Input: part model. Units: mm. Frame: model coordinates. A direction names the side the tool comes from. Round coordinates to 2 decimals unless told otherwise and drop trailing zeros. Order: outer loops, then holes, each group sorted by start corner. A loop starts at its lowest first (then second) coordinate and runs counter-clockwise, first axis right, second up.
Item 1: Mould query, pull axis Z, two halves, no side actions, for faces 1 (the cylindrical face through (-1.984, 5.423, -1.521)), 2 (the flat face through (2, 0, -2)), 3 (the cylindrical face through (2.99, 18.45, -1.43)), 4 (the cylindrical face through (-0.867, 11.832, 3.905)). Classes: released by +Z, released by -Z, zero draft, split by the parting line, or undercut.
Item 2: Cut plane A-A on z = 0. Output: boundary loops of the cut face in (x, y), then the cut area to 3 significant figures.
Item 3: Cut plane C-C on x = 3. Output: boundary loops of the cut face in (y, z), then the cut area to 3 significant figures.
Item 4: Cut plane B-B on y = 18. Output: boundary loops of the cut face in (x, z).
Item 5: Line query: L1, parallel to Y at x = -3.6, z = 0; L2, parallel to X at y = 10, z = 0. Output: solid intervals per line, ascending.
Item 6: First-contact query: pin 1 (2.5 mm diameter, centred on x = 0, z = -0.5, fed in from -Y); pin 2 (1.8 mm diameter, centred on y = 18, z = 0, fed in from +X); pin 3 (1.5 mm diameter, centred on y = 5, z = -2, fed in from +X); pin 4 (2 mm diameter, centred on y = 19, z = -1, fed in from -X). Flat tips, straight axial feed; report the tip coordinate or a pass-through.
Item 7: Reachability of faces 5 (the cylindrical face through (2.99, 6.45, -1.43)), 6 (the flat face through (0, 11, 0)), 7 (the flat face through (0, 13, 0)) from +Z, -Z, +X, -X, +Y, -Y: full face, straight path, thin tool, end or side. Return the list, or none.
Item 8: Cut plane D-D on y = 3. Output: boundary loops of the cut face in (x, z), then the cut area to 3 significant figures.
```python
from build123d import *

# Parameters (mm, degrees)
SKETCH1_R               = 4
BOSS_EXTRUDE1_DEPTH     = 24
SKETCH2_R               = 2.5
CUT_EXTRUDE1_DEPTH      = 11
SKETCH3_R               = 2.5
CUT_EXTRUDE2_DEPTH      = 11
SKETCH4_R               = 1.5
CUT_EXTRUDE3_DEPTH      = 11
CUT_EXTRUDE3_DEPTH_BACK = 11


with BuildPart() as part:
    # Sketch1 → Boss-Extrude1 (new body)
    with BuildSketch(Plane(origin=(0, 0, 0), x_dir=(1, 0, 0), z_dir=(0, 1, 0))):
        Circle(SKETCH1_R)
    extrude(amount=BOSS_EXTRUDE1_DEPTH)

    # Sketch2 → Cut-Extrude1 (cut)
    with BuildSketch(Plane(origin=(0, 24, 0), x_dir=(1, 0, 0), z_dir=(0, 1, 0))):
        Circle(SKETCH2_R)
    extrude(amount=-CUT_EXTRUDE1_DEPTH, mode=Mode.SUBTRACT)

    # Sketch3 → Cut-Extrude2 (cut)
    with BuildSketch(Plane.XZ):
        Circle(SKETCH3_R)
    extrude(amount=-CUT_EXTRUDE2_DEPTH, mode=Mode.SUBTRACT)

    # Sketch4 → Cut-Extrude3 (cut, two sides)
    with BuildSketch(Plane(origin=(0, 0, 0), x_dir=(0, 0, -1), z_dir=(1, 0, 0))) as cut_extrude3_sk:
        with Locations((0, 18)):
            Circle(SKETCH4_R)
        with Locations((0, 6)):
            Circle(SKETCH4_R)
    extrude(amount=CUT_EXTRUDE3_DEPTH, mode=Mode.SUBTRACT)
    extrude(cut_extrude3_sk.sketch, amount=-CUT_EXTRUDE3_DEPTH_BACK, mode=Mode.SUBTRACT)


solid = part.part
```
From the geometry:
1. face 1: undercut
1. face 2: zero draft
1. face 3: undercut
1. face 4: split by the parting line
2. outline: (-4, 0) - (-2.5, 0) - (-2.5, 4.5) - (-4, 4.5) - close; (-4, 7.5) - (-2.5, 7.5) - (-2.5, 11) - (2.5, 11) - (2.5, 7.5) - (4, 7.5) - (4, 16.5) - (2.5, 16.5) - (2.5, 13) - (-2.5, 13) - (-2.5, 16.5) - (-4, 16.5) - close; (-4, 19.5) - (-2.5, 19.5) - (-2.5, 24) - (-4, 24) - close; (2.5, 0) - (4, 0) - (4, 4.5) - (2.5, 4.5) - close; (2.5, 19.5) - (4, 19.5) - (4, 24) - (2.5, 24) - close
2. area: 64.0 mm2
3. outline: (0, -2.65) - (24, -2.65) - (24, 2.65) - (0, 2.65) - close; hole circle Ø3 at (6, 0); hole circle Ø3 at (18, 0)
3. area: 113 mm2
4. outline: (-3.71, -1.5) arc R4 ccw to (3.71, -1.5) - (2, -1.5) arc R2.5 cw to (-2, -1.5) - close; (-3.71, 1.5) - (-2, 1.5) arc R2.5 cw to (2, 1.5) - (3.71, 1.5) arc R4 ccw to start
5. L1: y = 0 to 4.5, 7.5 to 16.5, 19.5 to 24
5. L2: x = -4 to -2.5, 2.5 to 4
6. pin 1: stops at y = 11
6. pin 2: passes through
6. pin 3: stops at x = 3.8
6. pin 4: stops at x = -4
7. face 5: +X, -X
7. face 6: -Y
7. face 7: +Y
8. outline: circle Ø8 at (0, 0); hole circle Ø5 at (0, 0)
8. area: 30.6 mm2
